Geometry check sheet. Reference: the model listing, model coordinates, mm. A direction names the side the tool comes from. Round coordinates to 2 decimals unless told otherwise and drop trailing zeros. Loops run counter-clockwise (first coordinate to the right, second up) from the corner with the lowest first, then second, coordinate; pieces in that order, holes last. Notation, with made-up numbers: (36, 79.25) - (81, 79.25) arc R21 ccw to (81, 104.25) - close; hole circle Ø8 at (75, -16). An arc over 180 degrees is marked (long way). Answer in a Markdown table with one row per item. Add a question column.
```python
from build123d import *

# Parameters (mm, degrees)
F1_DEPTH        = 9
F3_DEPTH        = 3
F4_R            = 8
F5_DEPTH        = 6
F5_DEPTH_BACK   = 17.5
F6_DEPTH        = 17.5
F7_R            = 8
F8_DEPTH        = 17.5
F8_DEPTH_BACK   = 6
F9_DEPTH        = 17.5
F11_D           = 3
F11_CSINK_D     = 8
F11_CSINK_ANGLE = 90


with BuildPart() as f1:
    # F0 (on Top) → F1 (new body)
    with BuildSketch(Plane.XY):
        Polygon((-15, -10), (-15, -27.5), (0, -27.5), (0, 0), (0, 27.5), (-15, 27.5), (-15, 10), (-7, 10), (-7, 0), (-7, -10), align=None)
        Polygon((0, 0), (0, -27.5), (15, -27.5), (15, 0), (15, 27.5), (0, 27.5), align=None)
    extrude(amount=-F1_DEPTH)

    # F2 (on face) → F3 (cut)
    with BuildSketch(Plane(origin=(0, 0, -9), x_dir=(1, 0, 0), z_dir=(0, 0, -1))):
        Polygon((-13, 25.5), (-13, 12), (-7, 12), (-5, 12), (-5, 10), (-5, -10), (-5, -12), (-7, -12), (-13, -12), (-13, -25.5), (13, -25.5), (13, 25.5), align=None)
    extrude(amount=-F3_DEPTH, mode=Mode.SUBTRACT)

    # F4 (on face) → F5 (join, two sides)
    with BuildSketch(Plane.XZ.offset(27.5)) as f5_sk:
        with BuildLine():
            ThreePointArc((-18.172145319, -7.7281751464), (-15.8238906872, -4.1769365873), (-15, 0))
            ThreePointArc((-15, 0), (-36.1761093128, 4.1769365873), (-18.172145319, -7.7281751464))
        make_face()
        with Locations((-26, 0)):
            Circle(F4_R, mode=Mode.SUBTRACT)
    extrude(amount=F5_DEPTH)
    extrude(f5_sk.sketch, amount=-F5_DEPTH_BACK)

    # F4 (on face) → F6 (join)
    with BuildSketch(Plane.XZ.offset(27.5)):
        with BuildLine():
            Line((-15, -9), (-15, 0))
            ThreePointArc((-15, 0), (-15.8238906872, -4.1769365873), (-18.172145319, -7.7281751464))
            Line((-18.172145319, -7.7281751464), (-15, -9))
        make_face()
    extrude(amount=-F6_DEPTH)

    # F7 (on face) → F8 (join, two sides)
    with BuildSketch(Plane(origin=(0, 27.5, 0), x_dir=(-1, 0, 0), z_dir=(0, 1, 0))) as f8_sk:
        with BuildLine():
            ThreePointArc((18.0354576911, -7.5872304439), (30.0859536587, -10.2129810878), (37, 0))
            ThreePointArc((37, 0), (26, 11), (15, 0))
            ThreePointArc((15, 0), (15.7870189122, -4.0859536587), (18.0354576911, -7.5872304439))
        make_face()
        with Locations((26, 0)):
            Circle(F7_R, mode=Mode.SUBTRACT)
    extrude(amount=-F8_DEPTH)
    extrude(f8_sk.sketch, amount=F8_DEPTH_BACK)

    # F7 (on face) → F9 (join)
    with BuildSketch(Plane(origin=(0, 27.5, 0), x_dir=(-1, 0, 0), z_dir=(0, 1, 0))):
        with BuildLine():
            ThreePointArc((18.0354576911, -7.5872304439), (15.7870189122, -4.0859536587), (15, 0))
            Line((15, 0), (15, -9))
            Line((15, -9), (18.0354576911, -7.5872304439))
        make_face()
    extrude(amount=-F9_DEPTH)

    # F11 (through all)
    with Locations(Plane.XY):
        with Locations((1, 18.5), (1, -18.5)):
            CounterSinkHole(F11_D / 2, F11_CSINK_D / 2, counter_sink_angle=F11_CSINK_ANGLE)


solid = f1.part
```
Q1. Cross-section at C-C, the plane z = 4.25. Enter the section's corners in (x, y), plus the area to 3 significant figures.
Q2. Cross-section at B-B, the plane x = -26. Enter the section's corners in (y, z), plus the area to 3 significant figures.
Q3. Scan lines: line 1 (Y direction, x = 1, z = -3.45); line 2 (Z direction, x = -26, y = 32.2); line 3 (Y direction, x = 0.5, z = -1.75). Record each from-to range of solid material in increasing order. Write a range as from..to.
Q4. Cross-section at A-A, the plane y = 18.5. Enter the section's corners in (x, z), plus the area to 3 significant figures.
Q5. Cross-section at D-D, the plane z = -3.5. Enter the section's corners in (x, y), plus the area to 3 significant figures.
Q6. Release check for a two-part mould opening along Y. For faces 6 (the flat face through (-24, 33.5, -8)), 7 (the flat face through (15, 0, -4)), 8 (the flat face through (-17, 10, -1)) record: +Y half, -Y half, draft (parallel to the pull), parting line (faces both ways), or undercut.
Q7. Depth check by flat-ended pin: P1, Ø5, axis at y = -6.5, z = 6.5, coming from the -X side; P2, Ø2.5, axis at x = -1, z = -8, coming from the -Y side; P3, Ø4.5, axis at x = -9, z = -4.5, coming from the +Y side; P4, Ø1, axis at x = -14, y = 25.5, coming from the +Z side. Enter the tip coordinate at first touch or a pass-through.
Q8. Set-up check for faces 1 (the flat face through (0, 0, 0)), 2 (the flat face through (-16.608, -18.873, -8.355)), 3 (the flat face through (-7, 0, -4)), 4 (the flat face through (-6, 0, -9)), 5 (the flat face through (-13, -19, -8)): record each of +Z, -Z, +X, -X, +Y, -Y from which the full face is reachable in a straight line by a thin tool's end or side.
Check sheet entries:
| question | item | result |
|---|---|---|
| 1 | outline | (-36.15, -33.5) - (-32.78, -33.5) - (-32.78, -10) - (-36.15, -10) - close; (-36.15, 10) - (-32.78, 10) - (-32.78, 33.5) - (-36.15, 33.5) - close; (-19.22, -33.5) - (-15.85, -33.5) - (-15.85, -10) - (-19.22, -10) - close; (-19.22, 10) - (-15.85, 10) - (-15.85, 33.5) - (-19.22, 33.5) - close |
| 1 | area | 317 mm² |
| 2 | outline | (-33.5, -11) - (-10, -11) - (-10, -8) - (-33.5, -8) - close; (-33.5, 8) - (-10, 8) - (-10, 11) - (-33.5, 11) - close; (10, -11) - (33.5, -11) - (33.5, -8) - (10, -8) - close; (10, 8) - (33.5, 8) - (33.5, 11) - (10, 11) - close |
| 2 | area | 282 mm² |
| 3 | line 1 | -27.5..-20, -17..17, 20..27.5 |
| 3 | line 2 | -11..-8, 8..11 |
| 3 | line 3 | -27.5..-20.69, -16.31..16.31, 20.69..27.5 |
| 4 | outline | (-18.04, -7.59) - (-15, -9) - (-13, -9) - (-13, -6) - (-0.5, -6) - (-0.5, -2.5) - (-3, 0) - (-15, 0) arc R11 ccw (long way) to start; (2.5, -6) - (13, -6) - (13, -9) - (15, -9) - (15, 0) - (5, 0) - (2.5, -2.5) - close; hole circle Ø16 at (-26, 0) |
| 4 | area | 356 mm² |
| 5 | outline | (-36.43, -33.5) - (-33.19, -33.5) - (-33.19, -10) - (-36.43, -10) - close; (-36.43, 10) - (-33.19, 10) - (-33.19, 33.5) - (-36.43, 33.5) - close; (-18.81, -33.5) - (-15.57, -33.5) - (-15.57, -27.5) - (15, -27.5) - (15, 27.5) - (-15.57, 27.5) - (-15.57, 33.5) - (-18.81, 33.5) - (-18.81, 10) - (-7, 10) - (-7, -10) - (-18.81, -10) - close; hole circle Ø3 at (1, -18.5); hole circle Ø3 at (1, 18.5) |
| 5 | area | 1,800 mm² |
| 6 | face 6 | +Y half |
| 6 | face 7 | draft |
| 6 | face 8 | undercut |
| 7 | P1 | through |
| 7 | P2 | y = -27.5 |
| 7 | P3 | y = 27.5 |
| 7 | P4 | z = 0 |
| 8 | face 1 | +Z, +X, +Y, -Y |
| 8 | face 2 | -Z, +Y, -Y |
| 8 | face 3 | +Z, -Z, -X |
| 8 | face 4 | -Z, +X, +Y, -Y |
| 8 | face 5 | -Z |
